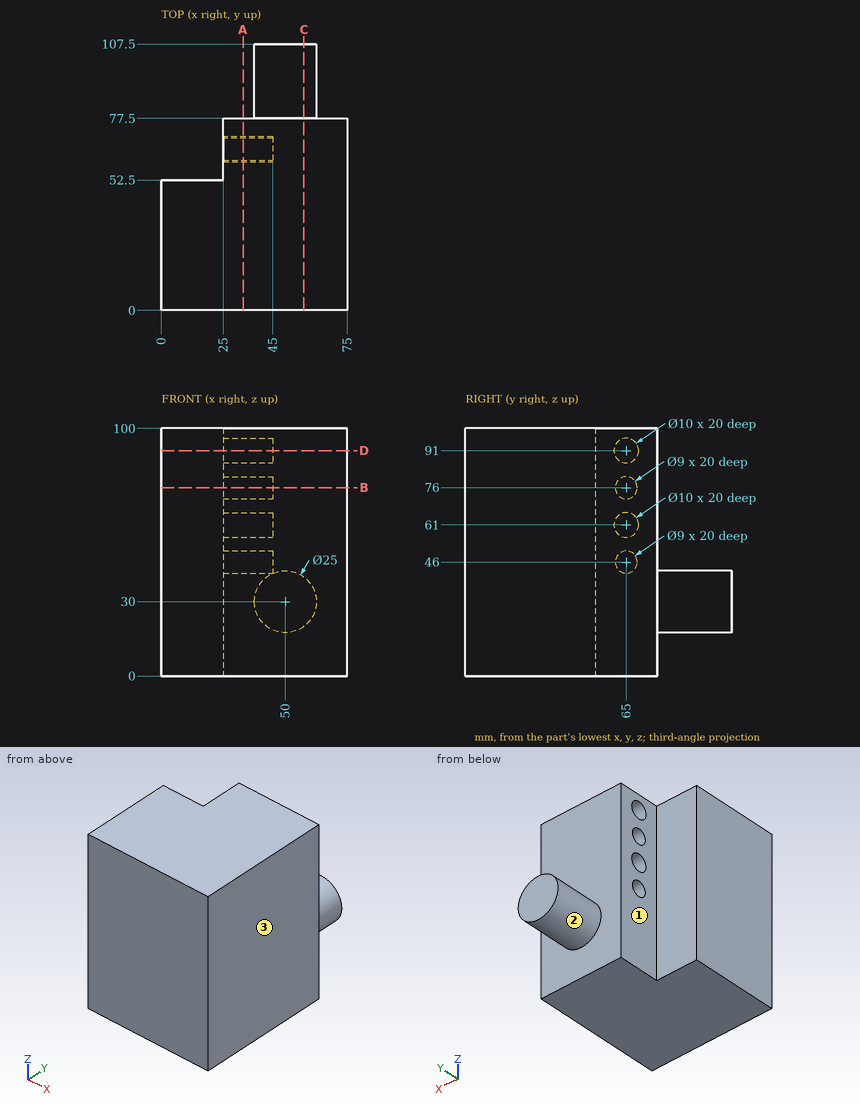
Geometry: see drawing. Coordinates: mm, zero at the bounding-box minimum. A direction names the side the tool comes from. Give positions to 0.01 mm unless a question says otherwise; leave off trailing zeros. Order: outer loops, then holes, each group sorted by start corner. A loop starts at its lowest first (then second) coordinate and runs counter-clockwise, first axis right, second up. Notation, with made-up numbers: (-22, -35.5) -> (13, -35.5) arc R24 cw to (13, -2.5) -> close; hole circle Ø10 at (-39, 49). An arc over 180 degrees is marked (long way). Write each question's results on one line, items separated by ' | '.
1) Cut plane B-B (z = 76). Output: boundary loops of the cut face in (x, y), and give its area (3 significant figures).
Geometry says:
outline: (0, 0) -> (75, 0) -> (75, 77.5) -> (25, 77.5) -> (25, 69.5) -> (45, 69.5) -> (45, 60.5) -> (25, 60.5) -> (25, 52.5) -> (0, 52.5) -> close | area: 5,010 mm²
2) Set-up query: the marked faces 1, 2 and 3. Return all of +Z, -Z, +X, -X, +Y, -Y with unobstructed straight access to the full face (end or side cutting, diameter ignored); none if empty.
Geometry says:
face 1: +Z, -Z, -X, +Y | face 2: +Y | face 3: +Z, -Z, +X, +Y, -Y
3) First-contact query: pin 1 Ø3 at (x, y) = (20, 41) entering from -Z; pin 2 Ø1 at (x, z) = (50, 87.5) entering from +Y; pin 3 Ø11.5 at (y, z) = (65, 76) entering from -X; pin 4 Ø6 at (x, y) = (35.5, 94.5) entering from -Z. Flat tips, straight axial feed; report the tip coordinate or a pass-through.
Geometry says:
pin 1: stops at z = 0 | pin 2: stops at y = 77.5 | pin 3: stops at x = 25 | pin 4: stops at z = 25.1
4) Cut plane C-C (x = 57.5). Output: boundary loops of the cut face in (y, z), and give its area (3 significant figures).
Geometry says:
outline: (0, 0) -> (77.5, 0) -> (77.5, 20) -> (107.5, 20) -> (107.5, 40) -> (77.5, 40) -> (77.5, 100) -> (0, 100) -> close | area: 8,350 mm²
5) Cut plane D-D (z = 91). Output: boundary loops of the cut face in (x, y).
Geometry says:
outline: (0, 0) -> (75, 0) -> (75, 77.5) -> (25, 77.5) -> (25, 70) -> (45, 70) -> (45, 60) -> (25, 60) -> (25, 52.5) -> (0, 52.5) -> close
6) Cut plane A-A (x = 33). Output: boundary loops of the cut face in (y, z), and give its area (3 significant figures).
Geometry says:
outline: (0, 0) -> (77.5, 0) -> (77.5, 100) -> (0, 100) -> close; hole circle Ø10 at (65, 61); hole circle Ø10 at (65, 91); hole circle Ø9 at (65, 46); hole circle Ø9 at (65, 76) | area: 7,470 mm²
7) Line query: line 1 along Z through (x, y) = (31.5, 65); line 2 along Y through (x, z) = (71, 61.5); line 3 along Y through (x, z) = (7, 37). Output: solid intervals per line, ascending.
Geometry says:
line 1: z = 0 to 41.5, 50.5 to 56, 66 to 71.5, 80.5 to 86, 96 to 100 | line 2: y = 0 to 77.5 | line 3: y = 0 to 52.5
